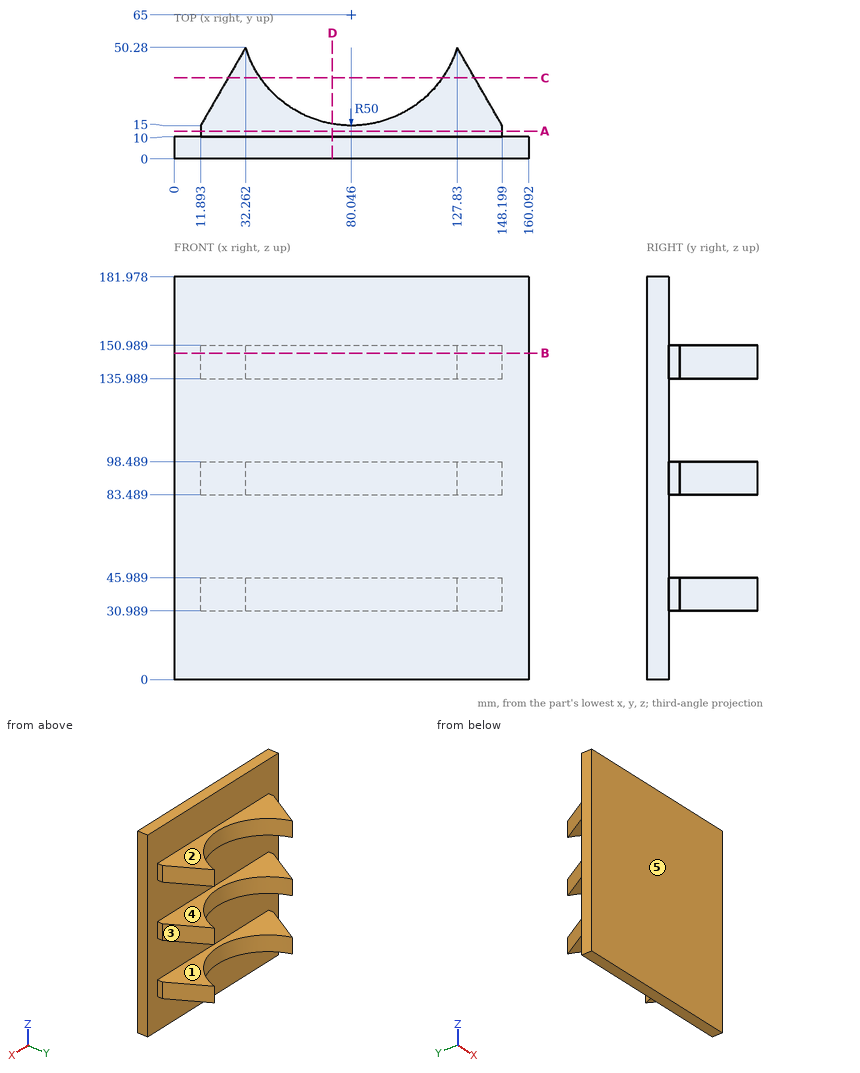
Can you work these out from the drawing? Everything is in mm from the part's minimum corner. A direction names the side the tool comes from. Give positions to 0.01 mm unless a question says otherwise; leave off trailing zeros. Order: outer loops, then holes, each group sorted by start corner. A loop starts at its lowest first (then second) coordinate and runs counter-clockwise, first axis right, second up. Notation, with made-up numbers: M 5,14.25 L 48,14.25 A16 ccw 48,31.25 Z; hole C -10.75,34.5 d2. An arc over 180 degrees is marked long. One line per item, written item: value.
Item 1: For the marked faces 4 and 5, which set-ups out of +Z, -Z, +X, -X, +Y, -Y let a thin tool reach every point of the face, with its end or its side?
Verdict:
face 4: +X, -X, +Y
face 5: +Z, -Z, +X, -X, -Y
Item 2: If we mould it in two halves opening along Z, with no side actions, what happens to the marked faces 1, 2 and 3? For each: pulls with the +Z half, pulls with the -Z half, needs draft (parallel to the pull), parting line crosses it, or undercut.
Verdict:
face 1: undercut
face 2: pulls with the +Z half
face 3: needs draft
Item 3: If we section it at C-C on y = 36.5: Write out the boundary of the cut face in (x, z).
Verdict:
outline: M 24.31,30.99 L 38.96,30.99 L 38.96,45.99 L 24.31,45.99 Z; M 24.31,83.49 L 38.96,83.49 L 38.96,98.49 L 24.31,98.49 Z; M 24.31,135.99 L 38.96,135.99 L 38.96,150.99 L 24.31,150.99 Z; M 121.13,30.99 L 135.79,30.99 L 135.79,45.99 L 121.13,45.99 Z; M 121.13,83.49 L 135.79,83.49 L 135.79,98.49 L 121.13,98.49 Z; M 121.13,135.99 L 135.79,135.99 L 135.79,150.99 L 121.13,150.99 Z
Item 4: If we section it at D-D on x = 71.5: Write out the boundary of the cut face in (y, z), and give its area (3 significant figures).
Verdict:
outline: M 0,0 L 10,0 L 10,30.99 L 15.74,30.99 L 15.74,45.99 L 10,45.99 L 10,83.49 L 15.74,83.49 L 15.74,98.49 L 10,98.49 L 10,135.99 L 15.74,135.99 L 15.74,150.99 L 10,150.99 L 10,181.98 L 0,181.98 Z
area: 2,080 mm2
Item 5: If we section it at A-A on y = 12.5: Write out the boundary of the cut face in (x, z), and give its area (3 significant figures).
Verdict:
outline: M 11.89,30.99 L 148.2,30.99 L 148.2,45.99 L 11.89,45.99 Z; M 11.89,83.49 L 148.2,83.49 L 148.2,98.49 L 11.89,98.49 Z; M 11.89,135.99 L 148.2,135.99 L 148.2,150.99 L 11.89,150.99 Z
area: 6,130 mm2
Item 6: Please list where these lines run through material, in increasing order: line 1 (Z direction, x = 126, y = 28); line 2 (Y direction, x = 87, z = 165); line 3 (X direction, y = 46, z = 95) (1 decimal).
Verdict:
line 1: 30.99 to 45.99, 83.49 to 98.49, 135.99 to 150.99
line 2: 0 to 10
line 3: 29.8 to 33.8, 126.3 to 130.3
Item 7: For pin 1 (6 mm diameter, centred on x = 19.5, z = 79.5, fed in from +Y); pin 2 (1.5 mm diameter, centred on x = 49, z = 160.5, fed in from -Y); pin 3 (20 mm diameter, centred on x = 83, y = 29.5, fed in from -Z); pin 4 (20 mm diameter, centred on x = 78, y = 22.5, fed in from +Z), each with a flat end and sliding along its axis, tell me the tip position at first contact or that it passes through.
Verdict:
pin 1: y = 10
pin 2: y = 0
pin 3: through
pin 4: z = 150.99
Item 8: If we section it at B-B on z = 147.5: Write out the boundary of the cut face in (x, y), and give its area (3 significant figures).
Verdict:
outline: M 0,0 L 160.09,0 L 160.09,10 L 148.2,10 L 148.2,15 L 127.83,50.28 A50 cw 32.26,50.28 L 11.89,15 L 11.89,10 L 0,10 Z
area: 3,900 mm2
